Verification items for the finished model (mm, model axes). Face numbers are marked on the shaded views. A direction names the side the tool comes from. Give positions to 0.01 mm unless a question says otherwise; leave off trailing zeros. Loops run counter-clockwise (first coordinate to the right, second up) from the corner with the lowest first, then second, coordinate; pieces in that order, holes last. Notation, with made-up numbers: (-39, -38) -> (13, -38) arc R29 ccw to (13, -7) -> close; hole circle Ø11 at (-7.75, 81). An arc over 180 degrees is marked (long way). Answer in a Markdown table with one row per item. Add a question column.
Q1. Section check A-A on x = -21.5. Enter the section's corners in (y, z), and give its area (3 significant figures).
Q2. Material ranges on probe 1 along Z at (x, y) = (23, 11); probe 2 along Z at (x, y) = (23, 4.75); probe 3 along X at (y, z) = (3.75, 5.25), recorded low to high.
Q3. Section check D-D on x = -4.5. Enter the section's corners in (y, z), and give its area (3 significant figures).
Q4. Set-up check for the marked faces 1, 2 and 3: record each of +Z, -Z, +X, -X, +Y, -Y from which the full face is reachable in a straight line by a thin tool's end or side.
Q5. Release check for a two-part mould opening along Z. For the marked faces 4, 5 and 6 record: pulls with the +Z half, pulls with the -Z half, needs draft (parallel to the pull), parting line crosses it, or undercut.
Q6. Gauge pin test, flat ends, axial feed: P1, Ø6, axis at x = 1.5, y = 7, coming from the +Z side; P2, Ø11.5, axis at x = -21.5, z = 9.5, coming from the -Y side; P3, Ø9, axis at x = 23, z = -3.5, coming from the -Y side; P4, Ø12, axis at x = -5, z = 12.5, coming from the +Y side. Record the tip position at first contact, or that the pin passes through.
Q7. Section check B-B on y = 7. Enter the section's corners in (x, z) (3 decimals), and give its area (3 significant figures).
Q8. Section check C-C on z = 3. Enter the section's corners in (x, y).
```python
from build123d import *

# Parameters (mm, degrees)
SKETCH1_W           = 57
SKETCH1_H           = 19
BOSS_EXTRUDE1_DEPTH = 15
SKETCH2_W           = 32
SKETCH2_H           = 1
CUT_EXTRUDE1_DEPTH  = 22
SKETCH3_R           = 5
CUT_EXTRUDE2_DEPTH  = 22
BOSS_EXTRUDE2_DEPTH = 6
SKETCH6_R           = 2.75
SKETCH6_R_2         = 2.5
CUT_EXTRUDE5_DEPTH  = 58.7
SKETCH8_R           = 5
CUT_EXTRUDE6_DEPTH  = 5.7
SKETCH9_R           = 8
CUT_EXTRUDE7_DEPTH  = 15.7
SKETCH10_R          = 5
CUT_EXTRUDE8_DEPTH  = 56.7
SKETCH11_R          = 8
BOSS_EXTRUDE3_DEPTH = 14
SKETCH12_R          = 5
BOSS_EXTRUDE4_DEPTH = 25
SKETCH13_R          = 8
CUT_EXTRUDE9_DEPTH  = 171
SKETCH14_R          = 5
CUT_EXTRUDE10_DEPTH = 171


with BuildPart() as part:
    # Sketch1 → Boss-Extrude1 (new body)
    with BuildSketch(Plane(origin=(0, 0, 0), x_dir=(1, 0, 0), z_dir=(0, 1, 0))):
        Rectangle(SKETCH1_W, SKETCH1_H)
    extrude(amount=BOSS_EXTRUDE1_DEPTH)

    # Sketch2 → Cut-Extrude1 (cut)
    with BuildSketch(Plane.XY.offset(9.5)):
        with Locations((1.5, 14.5)):
            Rectangle(SKETCH2_W, SKETCH2_H)
    extrude(amount=-CUT_EXTRUDE1_DEPTH, mode=Mode.SUBTRACT)

    # Sketch3 → Cut-Extrude2 (cut)
    with BuildSketch(Plane.XY.offset(9.5)):
        with Locations((0, 7)):
            Circle(SKETCH3_R)
    extrude(amount=-CUT_EXTRUDE2_DEPTH, mode=Mode.SUBTRACT)

    # Sketch5 → Boss-Extrude2 (add)
    with BuildSketch(Plane.XY.offset(9.5)):
        Polygon((-28.5, 15), (-14.5, 15), (-14.5, 14), (17.5, 14), (17.5, 15), (28.5, 15), (28.5, 0), (-28.5, 0), align=None)
    extrude(amount=BOSS_EXTRUDE2_DEPTH)

    # Sketch6 → Cut-Extrude5 (cut)
    with BuildSketch(Plane.XZ):
        with Locations((-21.5, 9.5)):
            Circle(SKETCH6_R)
        with Locations((23, -3.5)):
            Circle(SKETCH6_R)
        with Locations((-21.5, -3.5)):
            Circle(SKETCH6_R_2)
        with Locations((23, 9.5)):
            Circle(SKETCH6_R_2)
    extrude(amount=-CUT_EXTRUDE5_DEPTH, mode=Mode.SUBTRACT)

    # Sketch8 → Cut-Extrude6 (cut)
    with BuildSketch(Plane.XZ):
        with Locations((-21.5, 9.5)):
            Circle(SKETCH8_R)
        with Locations((23, -3.5)):
            Circle(SKETCH8_R)
    extrude(amount=-CUT_EXTRUDE6_DEPTH, mode=Mode.SUBTRACT)

    # Sketch9 → Cut-Extrude7 (cut)
    with BuildSketch(Plane.XZ):
        with Locations((0, 3)):
            Circle(SKETCH9_R)
    extrude(amount=-CUT_EXTRUDE7_DEPTH, mode=Mode.SUBTRACT)

    # Sketch10 → Cut-Extrude8 (cut)
    with BuildSketch(Plane(origin=(0, 0, -9.5), x_dir=(-1, 0, 0), z_dir=(0, 0, -1))):
        with Locations((0, 7)):
            Circle(SKETCH10_R)
    extrude(amount=-CUT_EXTRUDE8_DEPTH, mode=Mode.SUBTRACT)

    # Sketch11 → Boss-Extrude3 (add)
    with BuildSketch(Plane.XZ):
        with Locations((0, 3)):
            Circle(SKETCH11_R)
    extrude(amount=-BOSS_EXTRUDE3_DEPTH)

    # Sketch12 → Boss-Extrude4 (add)
    with BuildSketch(Plane.XY.offset(15.5)):
        with Locations((0, 7)):
            Circle(SKETCH12_R)
    extrude(amount=-BOSS_EXTRUDE4_DEPTH)

    # Sketch13 → Cut-Extrude9 (cut)
    with BuildSketch(Plane.XZ):
        with Locations((1.5, 3)):
            Circle(SKETCH13_R)
    extrude(amount=-CUT_EXTRUDE9_DEPTH, mode=Mode.SUBTRACT)

    # Sketch14 → Cut-Extrude10 (cut)
    with BuildSketch(Plane.XY.offset(15.5)):
        with Locations((1.5, 7)):
            Circle(SKETCH14_R)
    extrude(amount=-CUT_EXTRUDE10_DEPTH, mode=Mode.SUBTRACT)


solid = part.part
```
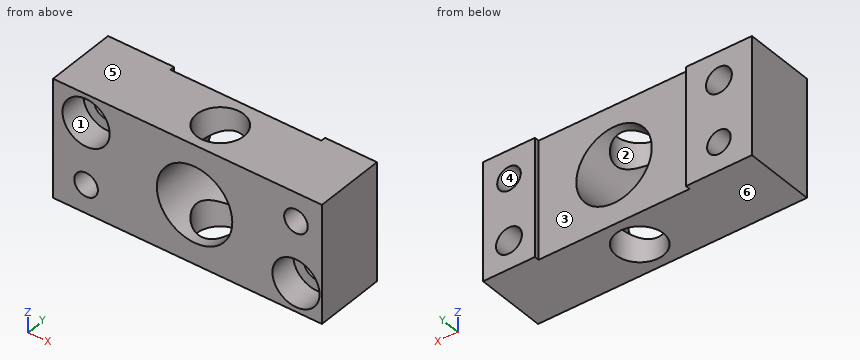
Taken from the geometry:
| question | item | result |
|---|---|---|
| 1 | outline | (0, -9.5) -> (15, -9.5) -> (15, -6) -> (0, -6) -> close; (0, -1) -> (15, -1) -> (15, 6.75) -> (5.7, 6.75) -> (5.7, 4.5) -> (0, 4.5) -> close; (0, 14.5) -> (5.7, 14.5) -> (5.7, 12.25) -> (15, 12.25) -> (15, 15.5) -> (0, 15.5) -> close |
| 1 | area | 192 mm² |
| 2 | probe 1 | z = -9.5 to -6.25, -0.75 to 7, 12 to 15.5 |
| 2 | probe 2 | z = -9.5 to -8.5, 1.5 to 7, 12 to 15.5 |
| 2 | probe 3 | x = -28.5 to -24.13, -18.87 to -6.18, 9.18 to 28.5 |
| 3 | outline | (0, -9.5) -> (14, -9.5) -> (14, -2.29) -> (0, -2.29) -> close; (0, 8.29) -> (14, 8.29) -> (14, 15.5) -> (0, 15.5) -> close |
| 3 | area | 202 mm² |
| 4 | face 1 | -Y |
| 4 | face 2 | +Z, -Z |
| 4 | face 3 | +Z, -Z, +Y |
| 5 | face 4 | undercut |
| 5 | face 5 | pulls with the +Z half |
| 5 | face 6 | pulls with the -Z half |
| 6 | P1 | passes through |
| 6 | P2 | stops at y = 0 |
| 6 | P3 | stops at y = 5.7 |
| 6 | P4 | stops at y = 14 |
| 7 | outline | (-28.5, -9.5) -> (-3.5, -9.5) -> (-3.5, -3.245) arc R8 cw to (-3.5, 9.245) -> (-3.5, 15.5) -> (-28.5, 15.5) -> close; (6.5, -9.5) -> (28.5, -9.5) -> (28.5, 15.5) -> (6.5, 15.5) -> (6.5, 9.245) arc R8 cw to (6.5, -3.245) -> close; hole circle Ø5.5 at (-21.5, 9.5); hole circle Ø5 at (-21.5, -3.5); hole circle Ø5.5 at (23, -3.5); hole circle Ø5 at (23, 9.5) |
| 7 | area | 1,040 mm² |
| 8 | outline | (-28.5, 0) -> (-6.5, 0) -> (-6.5, 14) -> (-14.5, 14) -> (-14.5, 15) -> (-28.5, 15) -> close; (9.5, 0) -> (28.5, 0) -> (28.5, 15) -> (17.5, 15) -> (17.5, 14) -> (9.5, 14) -> close |
